The model under review builds one solid part; all positions refer to its coordinate system, in mm. Face numbers are marked on the shaded views. A direction names the side the tool comes from. Round coordinates to 2 decimals unless told otherwise and drop trailing zeros. Write each loop counter-clockwise with the first axis right and the second up, starting at its lowest first coordinate (ties: lowest second). Pieces come first, ordered by that corner, then holes. Notation, with made-up numbers: (45, -16.75) -> (95, -16.75) arc R9 ccw to (95, -7.75) -> close; hole circle Ø7 at (21, 15). An arc over 180 degrees is marked (long way). Answer in a Markdown table with one row per item. Add a question column.
```python
from build123d import *

# Parameters (mm, degrees)
BOSS_EXTRUDE1_DEPTH = 115
CUT_EXTRUDE1_START  = -15
CUT_EXTRUDE1_DEPTH  = 15
BOSS_EXTRUDE2_START = -110
SKETCH3_W           = 20
SKETCH3_H           = 15
BOSS_EXTRUDE2_DEPTH = 120
SKETCH5_W           = 40
SKETCH5_H           = 33
CUT_EXTRUDE2_DEPTH  = 165.585219816
CUT_EXTRUDE3_DEPTH  = 139.495487291


with BuildPart() as part:
    # Sketch1 → Boss-Extrude1 (new body)
    with BuildSketch(Plane(origin=(0, 0, 0), x_dir=(1, 0, 0), z_dir=(0, 1, 0))):
        with BuildLine():
            Line((0, 0), (0, 25.362796982))
            Line((0, 25.362796982), (40, 25.362796982))
            Line((40, 25.362796982), (40, 40.362796982))
            Line((40, 40.362796982), (10, 40.362796982))
            Line((10, 40.362796982), (10, 106.362796982))
            ThreePointArc((10, 106.362796982), (-35.256322222, 56.96621079), (0, 0))
        make_face()
    extrude(amount=BOSS_EXTRUDE1_DEPTH)

    # Sketch2 → Cut-Extrude1 (cut)
    with BuildSketch(Plane(origin=(0, 115, 0), x_dir=(1, 0, 0), z_dir=(0, 1, 0)).offset(CUT_EXTRUDE1_START)):
        with BuildLine():
            Line((40, 30.362796982), (-35.235044142, 46.354499282))
            ThreePointArc((-35.235044142, 46.354499282), (-24.318751046, 85.179188449), (10, 106.362796982))
            Line((10, 106.362796982), (10, 40.362796982))
            Line((10, 40.362796982), (40, 40.362796982))
            Line((40, 40.362796982), (40, 30.362796982))
        make_face()
    extrude(amount=CUT_EXTRUDE1_DEPTH, mode=Mode.SUBTRACT)

    # Sketch3 → Boss-Extrude2 (add)
    with BuildSketch(Plane(origin=(0, 100, 0), x_dir=(1, 0, 0), z_dir=(0, 1, 0)).offset(BOSS_EXTRUDE2_START)):
        with Locations((5, 83.862796982)):
            Rectangle(SKETCH3_W, SKETCH3_H)
    extrude(amount=BOSS_EXTRUDE2_DEPTH)

    # Sketch5 → Cut-Extrude2 (cut, through all)
    with BuildSketch(Plane(origin=(15, 0, 0), x_dir=(0, 0, -1), z_dir=(1, 0, 0))):
        with Locations((86.362796982, 53.5)):
            Rectangle(SKETCH5_W, SKETCH5_H)
    extrude(amount=-CUT_EXTRUDE2_DEPTH, mode=Mode.SUBTRACT)

    # Sketch6 → Cut-Extrude3 (cut, through all)
    with BuildSketch(Plane(origin=(0, 0, -40.362796982), x_dir=(-1, 0, 0), z_dir=(0, 0, -1))):
        with BuildLine():
            Line((-25, 90), (-25, 10))
            ThreePointArc((-25, 10), (-30, 5), (-35, 10))
            Line((-35, 10), (-35, 90))
            ThreePointArc((-35, 90), (-30, 95), (-25, 90))
        make_face()
    extrude(amount=-CUT_EXTRUDE3_DEPTH, mode=Mode.SUBTRACT)


solid = part.part
```
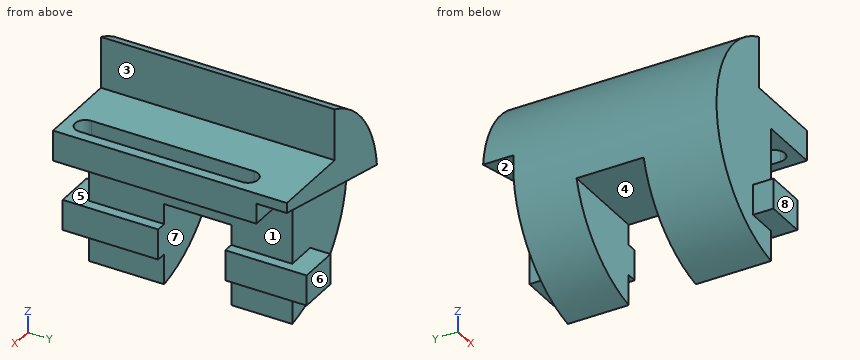
1. Add section C-C on z = -27.5. Write out the cut boundary in (x, y).
2. Mouldability with a two-part tool opening along Y and no side actions: class the marked faces 5, 6, 7 and 8 as pulls with the +Y half, pulls with the -Y half, needs draft (parallel to the pull), parting line crosses it, or undercut.
3. Insertion check: pin 1 Ø6 at (x, y) = (-15, 34.5) entering from +Z; pin 2 Ø8 at (y, z) = (41, -49.5) entering from +X; pin 3 Ø5 at (y, z) = (60, -18.5) entering from -X; pin 4 Ø6 at (x, z) = (3.5, -16.5) entering from +Y. Each pin has a flat end and moves straight along its axis. Give the tip position at first contact, or say it passes through.
4. Tool access review of the marked faces 1, 2, 3 and 4: name each direction out of +Z, -Z, +X, -X, +Y, -Y from which nothing blocks a thin tool from reaching the whole face with its end or side.
5. Add section B-B on x = 30. Write out the cut boundary in (y, z).
6. Add section D-D on y = 2. Write out the cut boundary in (x, z), plus the area to 3 significant figures.
7. For L1, parallel to Y at x = 4, z = -78.5; L2, parallel to Z at x = 17, y = 53.5; L3, parallel to Y at x = -21, z = -24.5, list the stretches that pass through material, from the lowest coordinate up.
8. Add section A-A on y = 39. Write out the cut boundary in (x, z).
Filled in:
| question | item | result |
|---|---|---|
| 1 | outline | (-29.91, 0) -> (40, 0) -> (40, 115) -> (-29.91, 115) -> close; hole (25, 10) arc R5 ccw to (35, 10) -> (35, 90) arc R5 ccw to (25, 90) -> close |
| 2 | face 5 | needs draft |
| 2 | face 6 | pulls with the +Y half |
| 2 | face 7 | undercut |
| 2 | face 8 | pulls with the -Y half |
| 3 | pin 1 | z = -6.43 |
| 3 | pin 2 | x = 10 |
| 3 | pin 3 | x = -26.19 |
| 3 | pin 4 | through |
| 4 | face 1 | +X, +Y, -Y |
| 4 | face 2 | +X, +Y |
| 4 | face 3 | +Z, +X, +Y, -Y |
| 4 | face 4 | -Z, +X, -X |
| 5 | outline | (0, -40.36) -> (5, -40.36) -> (5, -25.36) -> (0, -25.36) -> close; (95, -40.36) -> (100, -40.36) -> (100, -32.49) -> (115, -32.49) -> (115, -25.36) -> (95, -25.36) -> close |
| 6 | outline | (0, -25.36) -> (0, 0) arc R55.5 ccw to (10, -106.36) -> (10, -91.36) -> (15, -91.36) -> (15, -76.36) -> (10, -76.36) -> (10, -40.36) -> (40, -40.36) -> (40, -25.36) -> close |
| 6 | area | 3,990 mm² |
| 7 | L1 | -10 to 37, 70 to 110 |
| 7 | L2 | -40.36 to -25.36 |
| 7 | L3 | 0 to 115 |
| 8 | outline | (-33.55, -66.36) -> (10, -66.36) -> (10, -40.36) -> (25, -40.36) -> (25, -25.36) -> (0, -25.36) -> (0, 0) arc R55.5 ccw to start; (35, -40.36) -> (40, -40.36) -> (40, -25.36) -> (35, -25.36) -> close |
